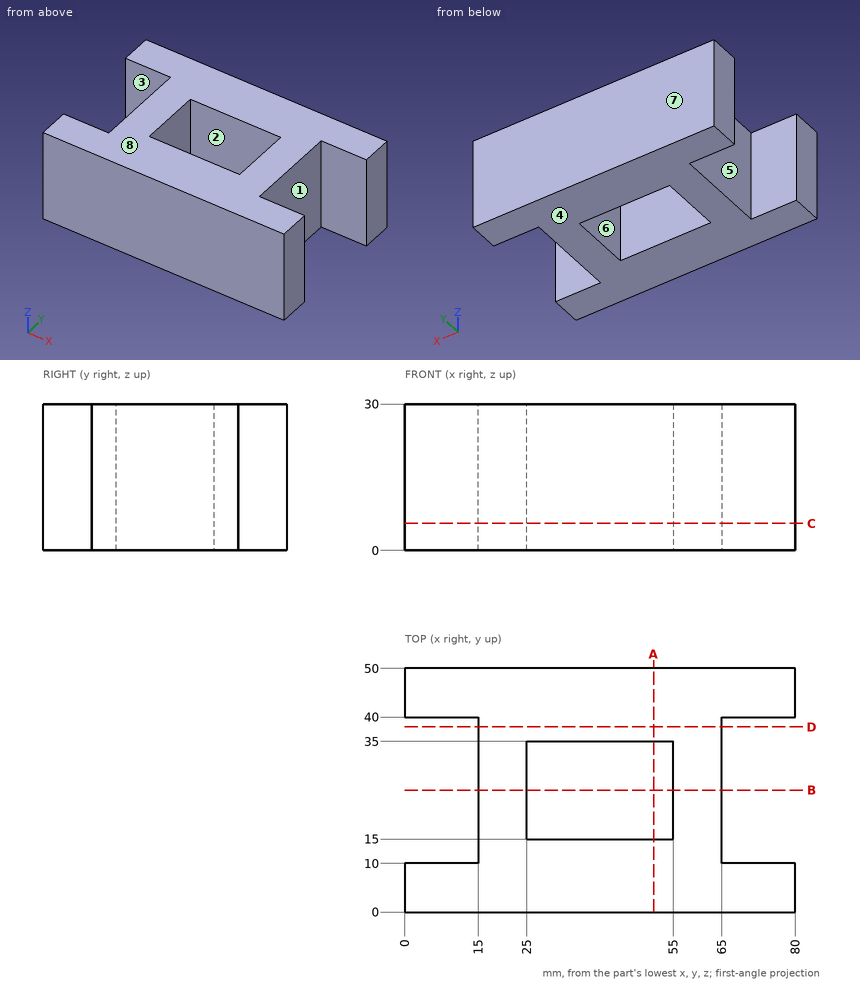
Study the drawing (mm; zero at the part's minimum x, y, z) and answer. A direction names the side the tool comes from. Coordinates: 2 decimals unless noted, no trailing zeros. Loops run counter-clockwise (first coordinate to the right, second up) from the corner with the lowest first, then second, coordinate; pieces in that order, holes last. Notation, with made-up numbers: M -22.5,37.25 L -0.5,37.25 A21 cw -0.5,41.25 Z; hole C -20.5,84 d11. An arc over 180 degrees is marked long. Answer in a Markdown table with one row per item. Add a question column.
1. Find section C-C, the plane z = 5.5. Write down the section's boundary in (x, y), then the cut area to 3 significant figures.
2. Flat-ended cylindrical pins translate along their axes: P1, Ø6, axis at y = 19, z = 23.5, coming from the -X side; P2, Ø6, axis at y = 33.5, z = 15, coming from the +X side. Find the tip coordinate at first contact, or state that the pin passes through.
3. Find section A-A, the plane x = 51. Write down the section's boundary in (y, z).
4. Find section B-B, the plane y = 25. Write down the section's boundary in (x, z).
5. Find section D-D, the plane y = 38. Write down the section's boundary in (x, z).
6. The mould has two halves that part along Y. Classify the marked faces 5, 6, 7 and 8: pulls with the +Y half, pulls with the -Y half, needs draft (parallel to the pull), parting line crosses it, or undercut.
7. A tool of negligible diameter and unlimited length cuts with its end or side. For the marked faces 1, 2, 3 and 4, from which of +Z, -Z, +X, -X, +Y, -Y can it reach the whole face along a straight path? Write none if from no direction.
8. Consider L1, parallel to X at y = 19.5, z = 28; L2, parallel to Y at x = 5, z = 28.5; L3, parallel to Y at x = 43, z = 20.25. Determine where each line is inside the solid, lowest interval first.
Reported:
| question | item | result |
|---|---|---|
| 1 | outline | M 0,0 L 80,0 L 80,10 L 65,10 L 65,40 L 80,40 L 80,50 L 0,50 L 0,40 L 15,40 L 15,10 L 0,10 Z; hole M 25,15 L 55,15 L 55,35 L 25,35 Z |
| 1 | area | 2,500 mm^2 |
| 2 | P1 | stops at x = 15 |
| 2 | P2 | stops at x = 65 |
| 3 | outline | M 0,0 L 15,0 L 15,30 L 0,30 Z; M 35,0 L 50,0 L 50,30 L 35,30 Z |
| 4 | outline | M 15,0 L 25,0 L 25,30 L 15,30 Z; M 55,0 L 65,0 L 65,30 L 55,30 Z |
| 5 | outline | M 15,0 L 65,0 L 65,30 L 15,30 Z |
| 6 | face 5 | undercut |
| 6 | face 6 | undercut |
| 6 | face 7 | pulls with the +Y half |
| 6 | face 8 | needs draft |
| 7 | face 1 | +Z, -Z, +X |
| 7 | face 2 | +Z, -Z |
| 7 | face 3 | +Z, -Z, -X |
| 7 | face 4 | -Z, +X, -X, +Y, -Y |
| 8 | L1 | x = 15 to 25, 55 to 65 |
| 8 | L2 | y = 0 to 10, 40 to 50 |
| 8 | L3 | y = 0 to 15, 35 to 50 |
